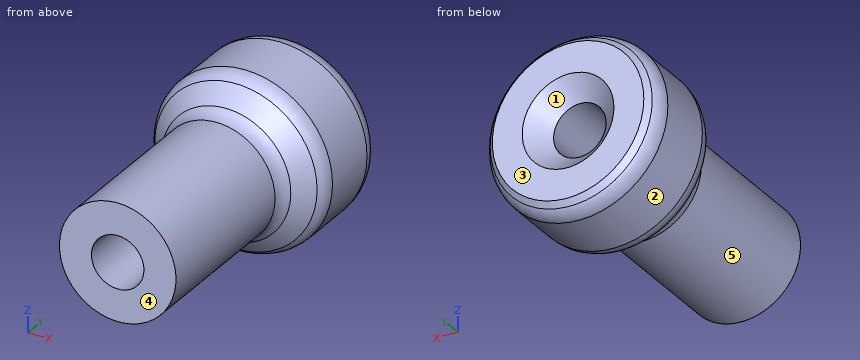
from build123d import *

# Parameters (mm, degrees)
SKETCH2_W                                       = 6
SKETCH2_H                                       = 6
SKETCH2_W_2                                     = 4
SKETCH2_H_2                                     = 14
CSK_FOR_M3_FLAT_HEAD_MACHINE_SCREW1_D           = 3.6
CSK_FOR_M3_FLAT_HEAD_MACHINE_SCREW1_CSINK_D     = 6.3
CSK_FOR_M3_FLAT_HEAD_MACHINE_SCREW1_CSINK_ANGLE = 90
CHAMFER1_SIZE                                   = 2
CHAMFER3_SIZE                                   = 0.8


with BuildPart() as part:
    # Sketch2 → Revolve1 (revolve)
    with BuildSketch(Plane.XY, mode=Mode.PRIVATE) as revolve1_sk:
        with Locations((3, 3)):
            Rectangle(SKETCH2_W, SKETCH2_H)
        with Locations((2, -7)):
            Rectangle(SKETCH2_W_2, SKETCH2_H_2)
    revolve(revolve1_sk.sketch.rotate(Axis((0, 0, 0), (0, -1, 0)), 180), axis=Axis((0, 0, 0), (0, -1, 0)))

    # CSK for M3 Flat Head Machine Screw1 (through all)
    with Locations(Plane(origin=(0, 6, 0), x_dir=(1, 0, 0), z_dir=(0, 1, 0))):
        with Locations((0, 0)):
            CounterSinkHole(CSK_FOR_M3_FLAT_HEAD_MACHINE_SCREW1_D / 2, CSK_FOR_M3_FLAT_HEAD_MACHINE_SCREW1_CSINK_D / 2, counter_sink_angle=CSK_FOR_M3_FLAT_HEAD_MACHINE_SCREW1_CSINK_ANGLE)

    # Chamfer1
    chamfer1_edges = [part.edges().sort_by_distance(p)[0] for p in [
        (4, 0, 0),
    ]]
    chamfer(chamfer1_edges, length=CHAMFER1_SIZE - 0.0001)  # a hair under: the kernel refuses the full size

    # Chamfer3
    chamfer3_edges = [part.edges().sort_by_distance(p)[0] for p in [
        (6, 6, 0),
    ]]
    chamfer(chamfer3_edges, length=CHAMFER3_SIZE)

    # Fillet1: read off the stored shape, not the designer's step
    # Fillet1 outline → Fillet1 (revolve, cut)
    with BuildSketch(Plane.XY):
        with BuildLine():
            ThreePointArc((5.560660172, 5.639339828), (5.885819299, 5.152704805), (6, 4.578679656))
            Line((6, 4.578679656), (6, 5.639339828))
            Line((6, 5.639339828), (5.560660172, 5.639339828))
        make_face()
        with BuildLine():
            Line((6, -0.439339828), (6, 0.621320344))
            ThreePointArc((6, 0.621320344), (5.885819299, 0.047295195), (5.560660172, -0.439339828))
            Line((5.560660172, -0.439339828), (6, -0.439339828))
        make_face()
    revolve(axis=Axis((0, 0, 0), (0, 1, 0)), mode=Mode.SUBTRACT)

    # Fillet1 2 outline → Fillet1 2 (revolve)
    with BuildSketch(Plane.XY):
        with BuildLine():
            ThreePointArc((4, -2.621320344), (4.114180701, -2.047295195), (4.439339828, -1.560660172))
            Line((4.439339828, -1.560660172), (4, -1.560660172))
            Line((4, -1.560660172), (4, -2.621320344))
        make_face()
    revolve(axis=Axis((0, 0, 0), (0, 1, 0)))


solid = part.part
Geometry check sheet. Reference: the model listing, model coordinates, mm. Face numbers are marked on the shaded views. A direction names the side the tool comes from. Give positions to 0.01 mm unless a question says otherwise; leave off trailing zeros. Write each loop counter-clockwise with the first axis right and the second up, starting at its lowest first coordinate (ties: lowest second). Pieces come first, ordered by that corner, then holes. Notation, with made-up numbers: M 52,34 L 74,34 A20 cw 74,44 Z; hole C 89,19 d3. An arc over 180 degrees is marked long. Answer as CSV lines item,"result". Start each with the question number.
Q1. Tool access check on the marked faces 4 and 5. Record the directions out of +Z, -Z, +X, -X, +Y, -Y that give a thin tool (end or side, any length) a straight path to the whole face; none if there is none.
Q2. Go/stop test with flat-tipped pins: pin 1 (4.5 mm diameter, centred on x = 0, z = 0, fed in from +Y); pin 2 (5 mm diameter, centred on y = -12, z = 4, fed in from -X); pin 3 (2 mm diameter, centred on y = -6.5, z = -3, fed in from +X). Record where each tip stops, or that it passes through.
Q3. Release check for a two-part mould opening along Z. For the marked faces 1, 2 and 3 record: pulls with the +Z half, pulls with the -Z half, needs draft (parallel to the pull), parting line crosses it, or undercut.
Q4. Section check C-C, the plane y = -6.25. Record the cut outline in (x, z), then the cut area to 3 significant figures.
Q5. Material ranges on L1, parallel to Z at x = 0, y = -3.5; L2, parallel to X at y = 1, z = 0.5; L3, parallel to X at y = 3.5, z = -0.25, recorded low to high.
Geometry says:
1,face 4,"+Z, -Z, +X, -X, -Y"
1,face 5,"-Y"
2,pin 1,"y = 5.1"
2,pin 2,"x = -3.71"
2,pin 3,"x = 3.46"
3,face 1,"undercut"
3,face 2,"parting line crosses it"
3,face 3,"needs draft"
4,outline,"C 0,0 d8; hole C 0,0 d3.6"
4,area,"40.1 mm^2"
5,L1,"-4 to -1.8, 1.8 to 4"
5,L2,"-5.98 to -1.73, 1.73 to 5.98"
5,L3,"-5.99 to -1.78, 1.78 to 5.99"
